Read the model definition and answer for the solid it produces. Units are mm, in the model's axes. A direction names the side the tool comes from. Coordinates: 2 decimals unless noted, no trailing zeros. Use CSV: the item, a comma, the result in double quotes.
```python
from build123d import *

# Parameters (mm, degrees)
F0_W      = 584.2
F0_H      = 596.9
F1_DEPTH  = 19.05
F2_R      = 9.525
F3_DEPTH  = 6.35
F4_R      = 3.9624
F5_DEPTH  = 19.051
F6_R      = 9.525
F7_DEPTH  = 6.35
F8_R      = 9.525
F9_DEPTH  = 1.905
F10_R     = 3.96875
F11_DEPTH = 19.051
F12_R     = 9.525
F13_DEPTH = 1.905


with BuildPart() as f1:
    # F0 (on Top) → F1 (new body)
    with BuildSketch(Plane.XY):
        with Locations((292.1, -298.45)):
            Rectangle(F0_W, F0_H)
    extrude(amount=F1_DEPTH)

    # F2 (on face) → F3 (cut)
    with BuildSketch(Plane.XY.offset(19.05)):
        with Locations((25.4, -552.45)):
            Circle(F2_R)
        with Locations((25.4, -44.45)):
            Circle(F2_R)
        with Locations((558.8, -552.45)):
            Circle(F2_R)
        with Locations((558.8, -44.45)):
            Circle(F2_R)
    extrude(amount=-F3_DEPTH, mode=Mode.SUBTRACT)

    # F4 (on face) → F5 (cut, through all)
    with BuildSketch(Plane.XY.offset(19.05)):
        with Locations((25.4, -552.45)):
            Circle(F4_R)
        with Locations((25.4, -44.45)):
            Circle(F4_R)
        with Locations((558.8, -552.45)):
            Circle(F4_R)
        with Locations((558.8, -44.45)):
            Circle(F4_R)
    extrude(amount=-F5_DEPTH, mode=Mode.SUBTRACT)

    # F6 (on face) → F7 (cut)
    with BuildSketch(Plane(origin=(0, 0, 0), x_dir=(1, 0, 0), z_dir=(0, 0, -1))):
        with Locations((25.4, 44.45)):
            Circle(F6_R)
        with Locations((25.4, 552.45)):
            Circle(F6_R)
        with Locations((558.8, 44.45)):
            Circle(F6_R)
        with Locations((558.8, 552.45)):
            Circle(F6_R)
    extrude(amount=-F7_DEPTH, mode=Mode.SUBTRACT)

    # F8 (on face) → F9 (cut)
    with BuildSketch(Plane.XY.offset(19.05)):
        with Locations((63.5, -552.45)):
            Circle(F8_R)
        with Locations((63.5, -450.85)):
            Circle(F8_R)
        with Locations((63.5, -349.25)):
            Circle(F8_R)
        with Locations((63.5, -247.65)):
            Circle(F8_R)
        with Locations((63.5, -146.05)):
            Circle(F8_R)
        with Locations((63.5, -44.45)):
            Circle(F8_R)
        with Locations((177.8, -552.45)):
            Circle(F8_R)
        with Locations((177.8, -450.85)):
            Circle(F8_R)
        with Locations((177.8, -349.25)):
            Circle(F8_R)
        with Locations((177.8, -247.65)):
            Circle(F8_R)
        with Locations((177.8, -146.05)):
            Circle(F8_R)
        with Locations((177.8, -44.45)):
            Circle(F8_R)
        with Locations((292.1, -552.45)):
            Circle(F8_R)
        with Locations((292.1, -450.85)):
            Circle(F8_R)
        with Locations((292.1, -349.25)):
            Circle(F8_R)
        with Locations((292.1, -247.65)):
            Circle(F8_R)
        with Locations((292.1, -146.05)):
            Circle(F8_R)
        with Locations((292.1, -44.45)):
            Circle(F8_R)
        with Locations((406.4, -552.45)):
            Circle(F8_R)
        with Locations((406.4, -450.85)):
            Circle(F8_R)
        with Locations((406.4, -349.25)):
            Circle(F8_R)
        with Locations((406.4, -247.65)):
            Circle(F8_R)
        with Locations((406.4, -146.05)):
            Circle(F8_R)
        with Locations((406.4, -44.45)):
            Circle(F8_R)
        with Locations((520.7, -552.45)):
            Circle(F8_R)
        with Locations((520.7, -450.85)):
            Circle(F8_R)
        with Locations((520.7, -349.25)):
            Circle(F8_R)
        with Locations((520.7, -247.65)):
            Circle(F8_R)
        with Locations((520.7, -146.05)):
            Circle(F8_R)
        with Locations((520.7, -44.45)):
            Circle(F8_R)
    extrude(amount=-F9_DEPTH, mode=Mode.SUBTRACT)

    # F10 (on face) → F11 (cut, through all)
    with BuildSketch(Plane.XY.offset(19.05)):
        with Locations((63.5, -552.45)):
            Circle(F10_R)
        with Locations((63.5, -450.85)):
            Circle(F10_R)
        with Locations((63.5, -349.25)):
            Circle(F10_R)
        with Locations((63.5, -247.65)):
            Circle(F10_R)
        with Locations((63.5, -146.05)):
            Circle(F10_R)
        with Locations((63.5, -44.45)):
            Circle(F10_R)
        with Locations((177.8, -552.45)):
            Circle(F10_R)
        with Locations((177.8, -450.85)):
            Circle(F10_R)
        with Locations((177.8, -349.25)):
            Circle(F10_R)
        with Locations((177.8, -247.65)):
            Circle(F10_R)
        with Locations((177.8, -146.05)):
            Circle(F10_R)
        with Locations((177.8, -44.45)):
            Circle(F10_R)
        with Locations((292.1, -552.45)):
            Circle(F10_R)
        with Locations((292.1, -450.85)):
            Circle(F10_R)
        with Locations((292.1, -349.25)):
            Circle(F10_R)
        with Locations((292.1, -247.65)):
            Circle(F10_R)
        with Locations((292.1, -146.05)):
            Circle(F10_R)
        with Locations((292.1, -44.45)):
            Circle(F10_R)
        with Locations((406.4, -552.45)):
            Circle(F10_R)
        with Locations((406.4, -450.85)):
            Circle(F10_R)
        with Locations((406.4, -349.25)):
            Circle(F10_R)
        with Locations((406.4, -247.65)):
            Circle(F10_R)
        with Locations((406.4, -146.05)):
            Circle(F10_R)
        with Locations((406.4, -44.45)):
            Circle(F10_R)
        with Locations((520.7, -552.45)):
            Circle(F10_R)
        with Locations((520.7, -450.85)):
            Circle(F10_R)
        with Locations((520.7, -349.25)):
            Circle(F10_R)
        with Locations((520.7, -247.65)):
            Circle(F10_R)
        with Locations((520.7, -146.05)):
            Circle(F10_R)
        with Locations((520.7, -44.45)):
            Circle(F10_R)
    extrude(amount=-F11_DEPTH, mode=Mode.SUBTRACT)

    # F12 (on face) → F13 (cut)
    with BuildSketch(Plane(origin=(0, 0, 0), x_dir=(1, 0, 0), z_dir=(0, 0, -1))):
        with Locations((63.5, 552.45)):
            Circle(F12_R)
        with Locations((63.5, 450.85)):
            Circle(F12_R)
        with Locations((63.5, 349.25)):
            Circle(F12_R)
        with Locations((63.5, 247.65)):
            Circle(F12_R)
        with Locations((63.5, 146.05)):
            Circle(F12_R)
        with Locations((63.5, 44.45)):
            Circle(F12_R)
        with Locations((177.8, 552.45)):
            Circle(F12_R)
        with Locations((177.8, 450.85)):
            Circle(F12_R)
        with Locations((177.8, 349.25)):
            Circle(F12_R)
        with Locations((177.8, 247.65)):
            Circle(F12_R)
        with Locations((177.8, 146.05)):
            Circle(F12_R)
        with Locations((177.8, 44.45)):
            Circle(F12_R)
        with Locations((292.1, 552.45)):
            Circle(F12_R)
        with Locations((292.1, 450.85)):
            Circle(F12_R)
        with Locations((292.1, 349.25)):
            Circle(F12_R)
        with Locations((292.1, 247.65)):
            Circle(F12_R)
        with Locations((292.1, 146.05)):
            Circle(F12_R)
        with Locations((292.1, 44.45)):
            Circle(F12_R)
        with Locations((406.4, 552.45)):
            Circle(F12_R)
        with Locations((406.4, 450.85)):
            Circle(F12_R)
        with Locations((406.4, 349.25)):
            Circle(F12_R)
        with Locations((406.4, 247.65)):
            Circle(F12_R)
        with Locations((406.4, 146.05)):
            Circle(F12_R)
        with Locations((406.4, 44.45)):
            Circle(F12_R)
        with Locations((520.7, 552.45)):
            Circle(F12_R)
        with Locations((520.7, 450.85)):
            Circle(F12_R)
        with Locations((520.7, 349.25)):
            Circle(F12_R)
        with Locations((520.7, 247.65)):
            Circle(F12_R)
        with Locations((520.7, 146.05)):
            Circle(F12_R)
        with Locations((520.7, 44.45)):
            Circle(F12_R)
    extrude(amount=-F13_DEPTH, mode=Mode.SUBTRACT)


solid = f1.part
```
Item 1: Each of these flat-tipped pins is pushed along its axis until it touches: P1, Ø10.5, axis at x = 177.8, y = -349.25, coming from the -Z side (3 decimals); P2, Ø5.5, axis at x = 411, y = -349.5, coming from the +Z side (3 decimals); P3, Ø9.5, axis at x = 555, y = -550.5, coming from the +Z side. Where does it stop, or does it pass through?
Return value:
P1,"stops at z = 1.905"
P2,"stops at z = 17.145"
P3,"stops at z = 12.7"
Item 2: The mould has two halves that part along X. Classify faces 1 (the flat face through (288, -596.9, 9)), 2 (the flat face through (68, -146, 1.905)): +X half, -X half, draft (parallel to the pull), parting line (faces both ways), or undercut.
Return value:
face 1,"draft"
face 2,"undercut"
Item 3: A tool of negligible diameter and unlimited length cuts with its end or side. For faces 3 (the cylindrical face through (415.485, -47.311, 0.939)), 4 (the flat face through (292, -49, 17.145)), from which of +Z, -Z, +X, -X, +Y, -Y can it reach the whole face along a straight path? Write none if from no direction.
Return value:
face 3,"-Z"
face 4,"+Z"
Item 4: Straight lines are drawn through the part: line 1 along X through (y, z) = (-146.05, 0.8) (3 decimals); line 2 along X through (y, z) = (-40, 17). For each, find the intervals that lie inside material, in ascending order.
Return value:
line 1,"x = 0 to 53.975, 73.025 to 168.275, 187.325 to 282.575, 301.625 to 396.875, 415.925 to 511.175, 530.225 to 584.2"
line 2,"x = 0 to 16.98, 33.82 to 550.38, 567.22 to 584.2"
